from build123d import *

# Parameters (mm, degrees)
SKETCH1_R           = 2
SKETCH1_R_2         = 3
BOSS_EXTRUDE1_DEPTH = 5
SKETCH1_3_R         = 1.74625
BOSS_EXTRUDE2_DEPTH = 15
FILLET1_R           = 3


with BuildPart() as part:
    # Sketch1 → Boss-Extrude1 (new body)
    with BuildSketch(Plane.XY):
        with BuildLine():
            Line((10, -25.3), (10, -6.5))
            Line((10, -6.5), (-10, -6.5))
            Line((-10, -6.5), (-10, -25.3))
            ThreePointArc((-10, -25.3), (0, -35.3), (10, -25.3))
        make_face()
        with Locations((0, -25.3)):
            Circle(SKETCH1_R, mode=Mode.SUBTRACT)
        with Locations((0, -13)):
            Circle(SKETCH1_R_2, mode=Mode.SUBTRACT)
    extrude(amount=BOSS_EXTRUDE1_DEPTH)

    # Sketch1<3> → Boss-Extrude2 (add)
    with BuildSketch(Plane.XY):
        with BuildLine():
            Line((10, -6.5), (10, 0))
            ThreePointArc((10, 0), (0, 10), (-10, 0))
            Line((-10, 0), (-10, -6.5))
            Line((-10, -6.5), (10, -6.5))
        make_face()
        Circle(SKETCH1_3_R, mode=Mode.SUBTRACT)
    extrude(amount=BOSS_EXTRUDE2_DEPTH)

    # Fillet1
    fillet1_edges = [part.edges().sort_by_distance(p)[0] for p in [
        (-10, -6.5, 10),
        (10, -6.5, 10),
    ]]
    fillet(fillet1_edges, radius=FILLET1_R)


solid = part.part
Input: part model. Units: mm. Frame: model coordinates. A direction names the side the tool comes from. Coordinates: 2 decimals unless noted, no trailing zeros. Loops run counter-clockwise (first coordinate to the right, second up) from the corner with the lowest first, then second, coordinate; pieces in that order, holes last. Notation, with made-up numbers: (24.25, 17) - (37.25, 17) arc R11 ccw to (37.25, 32) - close; hole circle Ø5 at (-23, 64.25). An arc over 180 degrees is marked (long way). Answer in a Markdown table with one row per item. Add a question column.
Item 1: Line query: line 1 along Y through (x, z) = (0, 1); line 2 along Y through (x, z) = (0, 5.75); line 3 along Z through (x, y) = (-0.75, -7). Output: solid intervals per line, ascending. Write a range as [from, to].
Item 2: Access query for faces 1 (the cylindrical face through (9.14, -5.6, 10.07)), 2 (the flat face through (0, -6.5, 10)), 3 (the cylindrical face through (-9.14, -5.6, 10.07)). Directions: +Z, -Z, +X, -X, +Y, -Y. A direction counts if a zero-diameter tool reaches every point of the face in a straight line with its end or side. Return the directions, or none.
Item 3: Section query B-B on y = -13. Return the cut outline in (x, z), then the cut area to 3 significant figures.
Item 4: Contact query for flat-ended pins moving along their axis: P1, Ø4.5, axis at x = 0, y = 0, coming from the -Z side; P2, Ø4, axis at x = -6, z = 13, coming from the -Y side; P3, Ø3.5, axis at x = 0, y = -25.3, coming from the -Z side; P4, Ø1.5, axis at x = -7, z = 10.5, coming from the +Y side. Output: stop coordinate, or through.
Item 5: Section query A-A on x = 0. Return the cut outline in (y, z).
Item 6: Section query C-C on z = 2.5. Return the cut outline in (x, y), then the cut area to 3 significant figures.
Item 7: Mould query, pull axis X, two halves, no side actions, for faces 4 (the cylindrical face through (0, 10, 7)), 5 (the cylindrical face through (-0.434, -27.252, 2.465)), 6 (the cylindrical face through (-0.23, 1.73, 7.4)), 7 (the flat face through (10, -10, 4)). Classes: released by +X, released by -X, zero draft, split by the parting line, or undercut.
Item 8: Section query D-D on z = 10.5. Return the cut outline in (x, y).
Recorded:
| question | item | result |
|---|---|---|
| 1 | line 1 | [-35.3, -27.3], [-23.3, -16], [-10, -1.75], [1.75, 10] |
| 1 | line 2 | [-6.5, -1.75], [1.75, 10] |
| 1 | line 3 | [0, 5] |
| 2 | face 1 | +Z, +X, -Y |
| 2 | face 2 | +Z, +X, -X, -Y |
| 2 | face 3 | +Z, -X, -Y |
| 3 | outline | (-10, 0) - (-3, 0) - (-3, 5) - (-10, 5) - close; (3, 0) - (10, 0) - (10, 5) - (3, 5) - close |
| 3 | area | 70.0 mm^2 |
| 4 | P1 | z = 0 |
| 4 | P2 | y = -6.5 |
| 4 | P3 | through |
| 4 | P4 | y = 7.81 |
| 5 | outline | (-35.3, 0) - (-27.3, 0) - (-27.3, 5) - (-35.3, 5) - close; (-23.3, 0) - (-16, 0) - (-16, 5) - (-23.3, 5) - close; (-10, 0) - (-1.75, 0) - (-1.75, 15) - (-6.5, 15) - (-6.5, 5) - (-10, 5) - close; (1.75, 0) - (10, 0) - (10, 15) - (1.75, 15) - close |
| 6 | outline | (-10, -25.3) arc R10 ccw to (10, -25.3) - (10, 0) arc R10 ccw to (-10, 0) - close; hole circle Ø6 at (0, -13); hole circle Ø4 at (0, -25.3); hole circle Ø3.49 at (0, 0) |
| 6 | area | 770 mm^2 |
| 7 | face 4 | split by the parting line |
| 7 | face 5 | undercut |
| 7 | face 6 | undercut |
| 7 | face 7 | released by +X |
| 8 | outline | (-10, -3.5) arc R3 ccw to (-7, -6.5) - (7, -6.5) arc R3 ccw to (10, -3.5) - (10, 0) arc R10 ccw to (-10, 0) - close; hole circle Ø3.49 at (0, 0) |
